Autodesk Inventor part; units mm, degrees
ref_plane "YZ Plane" through (0, 0, 0) normal (1, 0, 0) x (0, 1, 0)
ref_plane "XZ Plane" through (0, 0, 0) normal (0, 1, 0) x (-1, 0, 0)
ref_plane "XY Plane" through (0, 0, 0) normal (0, 0, 1) x (1, 0, 0)
sketch "Sketch1" plane through (0, 0, 0) normal (0, 1, 0) x (-1, 0, 0)
  line L0 (0, 0) -> (2.35, 0)
  line L1 (2.35, 0) -> (2.65, 6.4)
  line L2 (2.65, 6.4) -> (14.45, 6.4)
  line L3 (14.45, 6.4) -> (14.75, 0)
  line L4 (14.75, 0) -> (17, 0)
  line L5 (17, 0) -> (17, -7)
  line L6 (17, -7) -> (15.75, -7)
  line L7 (15.75, -7) -> (15.75, -8.8)
  line L8 (15.75, -8.8) -> (17, -8.8)
  line L9 (17, -8.8) -> (17, -10.6)
  line L10 (17, -10.6) -> (20, -10.6)
  line L11 (20, -10.6) -> (20, -8.8)
  line L12 (20, -8.8) -> (21.25, -8.8)
  line L13 (21.25, -8.8) -> (21.25, -7)
  line L14 (21.25, -7) -> (20, -7)
  line L15 (20, -7) -> (20, 0)
  line L16 (20, 0) -> (25, 0)
  line L17 (25, 0) -> (25, -15)
  line L18 (25, -15) -> (0, -15)
  line L19 (0, -15) -> (0, 0)
  circle A0 centre (4.0344, -6.0871) radius 2.35
  dimension "d0" = 7
  dimension "d2" = 1.8
  dimension "d3" = 1.8
  dimension "d4" = 3
  dimension "d5" = 1.25
  dimension "d6" = 1.25
  dimension "d7" = 25
  dimension "d8" = 15
  dimension "d9" = 5
  dimension "d10" = 11.8
  dimension "d11" = 12.4
  dimension "d12" = 6.4
  dimension "d14" = 2.25
  dimension "d15" = 4.7
  dimension "d26" = 2.35
extrude "Extrusion1" add sketch "Sketch1" along normal blind 6.4
fillet "Fillet1" radius 2 2 edges at (-25, 3.2, -15) (0, 3.2, -15)
sketch "Sketch2" plane through (0, 6.4, 0) normal (0, 1, 0) x (1, 0, 0)
  line L0 (-25, 13) -> (-25, 0)
  line L1 (0, 0) -> (0, 13)
  circle A0 centre (-12.5, -10.4574) radius 25.0744
  line L2 (-25, 0) -> (-35.2897, 0)
  line L3 (-25, 0) -> (-25, 11.2791)
  line L4 (0, 0) -> (0, 11.2791)
  line L5 (0, 0) -> (10.2897, 0)
  dimension "d19" = 12.5
extrude "Extrusion2" add sketch "Sketch2" against normal blind 6.4 contours L0 L2 A0 | A0 L5 L1
sketch "Sketch3" plane through (0, 6.4, 0) normal (0, 1, 0) x (1, 0, 0)
  arc A0 (0, 13) -> (-2, 15) centre (-2, 13) ccw
  line L0 (-2, 15) -> (-23, 15)
  arc A1 (-23, 15) -> (-25, 13) centre (-23, 13) ccw
  line L1 (-25, 13) -> (-25, 11.2791)
  line L2 (0, 11.2791) -> (0, 13)
  circle A2 centre (-12.5, -10.4574) radius 25.0744
  point P0 (0, 0)
extrude "Extrusion3" cut sketch "Sketch3" against normal blind 6.4 contours L2 A2 L1 A1 L0 A0
sketch "Sketch4" plane through (0, 0, 0) normal (0, -1, 0) x (1, 0, 0)
  line L0 (10.2897, 0) -> (-2.35, 0)
  line L1 (-2.35, 0) -> (-2.65, 6.4)
  line L2 (-14.45, 6.4) -> (-14.75, 0)
  line L3 (-14.75, 0) -> (-17, 0)
  line L4 (-14.45, 6.4) -> (-14.65, 0)
  line L5 (-14.65, 0) -> (-14.75, 0)
  line L6 (-2.65, 6.4) -> (-2.45, 0)
  line L7 (-2.45, 0) -> (-2.35, 0)
  point P0 (0, 0)
  dimension "d27" = 0.1
  dimension "d28" = 0.1
extrude "Extrusion4" cut sketch "Sketch4" against normal blind 10
properties part number "trzymacz_bowdena"
Could you check a few things on this model? Use its own coordinates, in mm. A direction names the side the tool comes from. Give positions to 0.01 mm unless a question says otherwise; leave off trailing zeros. Write each loop counter-clockwise with the first axis right and the second up, starting at its lowest first coordinate (ties: lowest second). Pieces come first, ordered by that corner, then holes. Notation, with made-up numbers: (-39.75, 26) -> (-22.75, 26) arc R26 cw to (-22.75, 51) -> close; hole circle Ø1 at (-37.75, -35). An arc over 180 degrees is marked (long way). Answer as CSV lines item,"result". Start each with the question number.
(1) If we section it at A-A, the plane x = -16.5: Write out the boundary of the cut face in (y, z), and give its area (3 significant figures).
(2) Please list where these lines run through material, in increasing order: line 1 (X direction, y = 2, z = -6.25); line 2 (X direction, y = 1.25, z = -6.75); line 3 (Z direction, x = -13, y = 2.5).
(3) If we section it at D-D, the plane z = -5.25: Write out the boundary of the cut face in (x, y), and give its area (3 significant figures).
(4) Which directions (+Z, -Z, +X, -X, +Y, -Y) give clear straight access to the entire face, cutting with the end or side of a thin tool? Please do faces 1 (the face through (4, 3, 0)), 2 (the face through (-16, 3, 0)), 3 (the face through (-21.25, 3, -8)), 4 (the face through (-20, 3, -4)).
(5) If we mould it in two halves opening along X, with no side actions, what happens to faces 5 (the face through (-12, 6.4, -4)), 6 (the face through (-21, 3, -7))? For each: +X half, -X half, draft (parallel to the pull), parting line (faces both ways), or undercut.
(6) If we section it at C-C, the plane y = 4: Write out the boundary of the cut face in (x, z), and give its area (3 significant figures).
(7) If we section it at B-B, the plane z = -1: Write out the boundary of the cut face in (x, y).
(8) I'm going to push flat-ended pins straight in: pin 1 Ø1.4 at (y, z) = (1.5, -10) entering from -X; pin 2 Ø1.9 at (y, z) = (1.5, -4) entering from +X; pin 3 Ø0.6 at (x, y) = (-16.5, 3.5) entering from +Z. Where does each tip first touch, or does it pass through?
Answer list:
1,outline,"(0, -14.3) -> (6.4, -14.3) -> (6.4, -8.8) -> (0, -8.8) -> close; (0, -7) -> (6.4, -7) -> (6.4, 0) -> (0, 0) -> close"
1,area,"80.0 mm^2"
2,line 1,"-31.2 to -20, -17 to -6.38, -1.69 to 6.2"
2,line 2,"-30.74 to -20, -17 to -6.29, -1.78 to 5.74"
2,line 3,"-14.61 to 6.4"
3,outline,"(-32.04, 0) -> (-20, 0) -> (-20, 6.4) -> (-32.04, 6.4) -> close; (-17, 0) -> (-6.23, 0) -> (-6.23, 6.4) -> (-17, 6.4) -> close; (-1.84, 0) -> (7.04, 0) -> (7.04, 6.4) -> (-1.84, 6.4) -> close"
3,area,"203 mm^2"
4,face 1,"+Z, +X, +Y, -Y"
4,face 2,"+Z, -X, +Y, -Y"
4,face 3,"+Y, -Y"
4,face 4,"+Z, +Y, -Y"
5,face 5,"draft"
5,face 6,"undercut"
6,outline,"(-35.29, 0) arc R25.07 ccw to (10.29, 0) -> (-2.45, 0) -> (-2.65, 6.4) -> (-14.45, 6.4) -> (-14.65, 0) -> (-17, 0) -> (-17, -7) -> (-15.75, -7) -> (-15.75, -8.8) -> (-17, -8.8) -> (-17, -10.6) -> (-20, -10.6) -> (-20, -8.8) -> (-21.25, -8.8) -> (-21.25, -7) -> (-20, -7) -> (-20, 0) -> close; hole circle Ø4.7 at (-4.03, -6.09)"
6,area,"502 mm^2"
7,outline,"(-34.8, 0) -> (-20, 0) -> (-20, 6.4) -> (-34.8, 6.4) -> close; (-17, 0) -> (9.8, 0) -> (9.8, 6.4) -> (-17, 6.4) -> close"
8,pin 1,"x = -27.94"
8,pin 2,"x = 8.63"
8,pin 3,"z = 0"
